Drawing for the job (mm, zero at the part's lowest x, y, z). A direction names the side the tool comes from. Give positions to 0.01 mm unless a question says otherwise; leave off trailing zeros. Loops run counter-clockwise (first coordinate to the right, second up) from the corner with the lowest first, then second, coordinate; pieces in that order, holes last. Notation, with made-up numbers: (-2.75, -26) -> (35.25, -26) arc R22 cw to (35.25, -9) -> close; hole circle Ø6 at (84, 80.25). An arc over 180 degrees is marked (long way). Write item = value, one per line.
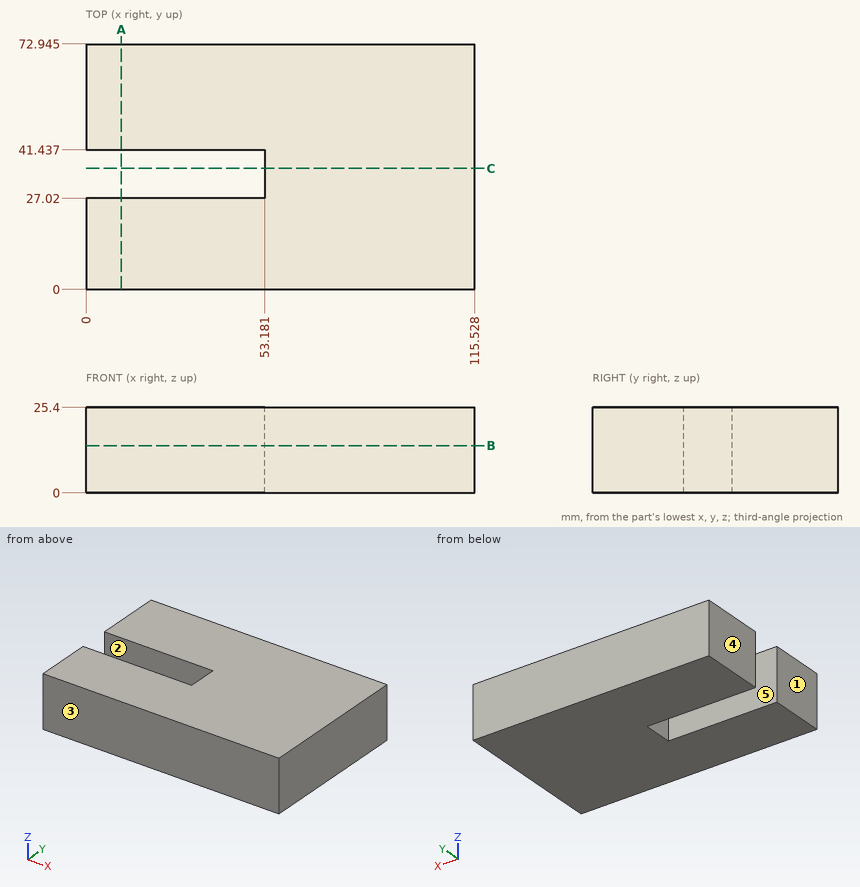
1) Pull direction Y, two halves, no side cores. Call the marked faces 3, 4 and 5: pulls with the +Y half, pulls with the -Y half, needs draft (parallel to the pull), parting line crosses it, or undercut.
Resolved:
face_3 = pulls with the -Y half
face_4 = needs draft
face_5 = undercut
2) Which spindle directions (+Z, -Z, +X, -X, +Y, -Y) get a long thin tool onto all of the face, cutting with end or side? Do the marked faces 1 and 2. Say none if no direction does.
Resolved:
face_1 = +Z, -Z, -X, +Y, -Y
face_2 = +Z, -Z, -X
3) Drop a flat-ended pin along its axis: P1, Ø1, axis at y = 40.5, z = 14.5, coming from the -X side. Give the stop position or say it passes through.
Resolved:
P1 = 53.18
4) Slice it at A-A, the plane x = 10.5. List the corners of the cut face in (y, z) (1 decimal).
Resolved:
outline = (0, 0) -> (27, 0) -> (27, 25.4) -> (0, 25.4) -> close; (41.4, 0) -> (72.9, 0) -> (72.9, 25.4) -> (41.4, 25.4) -> close
5) Slice it at B-B, the plane z = 14. List the corners of the cut face in (x, y) (1 decimal), and give its area (3 significant figures).
Resolved:
outline = (0, 0) -> (115.5, 0) -> (115.5, 72.9) -> (0, 72.9) -> (0, 41.4) -> (53.2, 41.4) -> (53.2, 27) -> (0, 27) -> close
area = 7,660 mm²
6) Slice it at C-C, the plane y = 36. List the corners of the cut face in (x, z), and give its area (3 significant figures).
Resolved:
outline = (53.18, 0) -> (115.53, 0) -> (115.53, 25.4) -> (53.18, 25.4) -> close
area = 1,580 mm²
7) Drill centre lines: line 1 along Y through (x, z) = (6, 5.5) (1 decimal); line 2 along X through (y, z) = (32.5, 6.75). Where is each one in solid material? Low to high. Write a range as [from, to].
Resolved:
line_1 = [0, 27], [41.4, 72.9]
line_2 = [53.18, 115.53]
